```python
from build123d import *

# Parameters (mm, degrees)
SKETCH2_R           = 13.5
BOSS_EXTRUDE2_DEPTH = 10
CUT_EXTRUDE1_DEPTH  = 59.489315264
BOSS_EXTRUDE3_DEPTH = 10
SKETCH5_R           = 1.7
CUT_EXTRUDE3_DEPTH  = 59.489315264


with BuildPart() as part:
    # Sketch2 → Boss-Extrude2 (new body)
    # profile 1 of 4: a face of its own
    with BuildSketch(Plane(origin=(0, 0, 0), x_dir=(1, 0, 0), z_dir=(0, 1, 0))):
        with BuildLine():
            ThreePointArc((4.652086817, 15.830606061), (3.552193091, 19.577649142), (0, 21.2))
            ThreePointArc((0, 21.2), (-3.552193091, 19.577649142), (-4.652086817, 15.830606061))
            ThreePointArc((-4.652086817, 15.830606061), (-3.188214551, 16.189048396), (-1.697742762, 16.412424242))
            ThreePointArc((-1.697742762, 16.412424242), (-0.043802421, 18.199435597), (1.7, 16.5))
            ThreePointArc((1.7, 16.5), (1.699435597, 16.456197579), (1.697742762, 16.412424242))
            ThreePointArc((1.697742762, 16.412424242), (3.188214551, 16.189048396), (4.652086817, 15.830606061))
        make_face()
    # profile 2 of 4: a face of its own
    with BuildSketch(Plane(origin=(0, 0, 0), x_dir=(1, 0, 0), z_dir=(0, 1, 0))):
        with BuildLine():
            ThreePointArc((-1.697742762, 16.412424242), (-3.188214551, 16.189048396), (-4.652086817, 15.830606061))
            ThreePointArc((-4.652086817, 15.830606061), (-16.5, 0), (-4.652086817, -15.830606061))
            ThreePointArc((-4.652086817, -15.830606061), (-3.188214551, -16.189048396), (-1.697742762, -16.412424242))
            ThreePointArc((-1.697742762, -16.412424242), (0, -14.8), (1.697742762, -16.412424242))
            ThreePointArc((1.697742762, -16.412424242), (3.188214551, -16.189048396), (4.652086817, -15.830606061))
            ThreePointArc((4.652086817, -15.830606061), (16.5, 0), (4.652086817, 15.830606061))
            ThreePointArc((4.652086817, 15.830606061), (3.188214551, 16.189048396), (1.697742762, 16.412424242))
            ThreePointArc((1.697742762, 16.412424242), (0, 14.8), (-1.697742762, 16.412424242))
        make_face()
        with Locations(Location((0, 0, 0), (0, 0, 270))):
            Circle(SKETCH2_R, mode=Mode.SUBTRACT)
    # profile 3 of 4: a face of its own
    with BuildSketch(Plane(origin=(0, 0, 0), x_dir=(1, 0, 0), z_dir=(0, 1, 0))):
        with BuildLine():
            ThreePointArc((-1.697742762, -16.412424242), (-3.188214551, -16.189048396), (-4.652086817, -15.830606061))
            ThreePointArc((-4.652086817, -15.830606061), (-3.552193091, -19.577649142), (0, -21.2))
            ThreePointArc((0, -21.2), (3.552193091, -19.577649142), (4.652086817, -15.830606061))
            ThreePointArc((4.652086817, -15.830606061), (3.188214551, -16.189048396), (1.697742762, -16.412424242))
            ThreePointArc((1.697742762, -16.412424242), (1.699435597, -16.456197579), (1.7, -16.5))
            ThreePointArc((1.7, -16.5), (-0.043802421, -18.199435597), (-1.697742762, -16.412424242))
        make_face()
    # profile 4 of 4: a face of its own
    with BuildSketch(Plane(origin=(0, 0, 0), x_dir=(1, 0, 0), z_dir=(0, 1, 0))):
        with BuildLine():
            Line((0, 36), (0, 21.2))
            ThreePointArc((0, 21.2), (3.552193091, 19.577649142), (4.652086817, 15.830606061))
            ThreePointArc((4.652086817, 15.830606061), (16.5, 0), (4.652086817, -15.830606061))
            ThreePointArc((4.652086817, -15.830606061), (3.552193091, -19.577649142), (0, -21.2))
            Line((0, -21.2), (0, -36))
            Line((0, -36), (45, -36))
            Line((45, -36), (45, 36))
            Line((45, 36), (0, 36))
        make_face()
    extrude(amount=BOSS_EXTRUDE2_DEPTH)

    # Sketch3 → Cut-Extrude1 (cut, through all)
    with BuildSketch(Plane(origin=(0, 10, 0), x_dir=(1, 0, 0), z_dir=(0, 1, 0))):
        with BuildLine():
            Line((3, 16.22498074), (3, 33))
            Line((3, 33), (42, 33))
            Line((42, 33), (42, -33))
            Line((42, -33), (3, -33))
            Line((3, -33), (3, -16.22498074))
            ThreePointArc((3, -16.22498074), (16.5, 0), (3, 16.22498074))
        make_face()
    extrude(amount=-CUT_EXTRUDE1_DEPTH, mode=Mode.SUBTRACT)

    # Sketch4 → Boss-Extrude3 (add, through all)
    with BuildSketch(Plane(origin=(0, 10, 0), x_dir=(1, 0, 0), z_dir=(0, 1, 0))):
        with BuildLine():
            Line((37, -33), (42, -33))
            Line((42, -33), (42, -28))
            ThreePointArc((42, -28), (38.464466094, -29.464466094), (37, -33))
        make_face()
        with BuildLine():
            Line((37, 33), (42, 33))
            Line((42, 33), (42, 28))
            ThreePointArc((42, 28), (38.464466094, 29.464466094), (37, 33))
        make_face()
    extrude(amount=-BOSS_EXTRUDE3_DEPTH)

    # Sketch5 → Cut-Extrude3 (cut, through all)
    with BuildSketch(Plane(origin=(0, 10, 0), x_dir=(1, 0, 0), z_dir=(0, 1, 0))):
        with Locations(Location((42, 33, 0), (0, 0, 270))):
            Circle(SKETCH5_R)
        with Locations(Location((42, -33, 0), (0, 0, 270))):
            Circle(SKETCH5_R)
    extrude(amount=-CUT_EXTRUDE3_DEPTH, mode=Mode.SUBTRACT)


solid = part.part
```
Verification items for the finished model (mm, model axes). A direction names the side the tool comes from. Coordinates: 2 decimals unless noted, no trailing zeros. Order: outer loops, then holes, each group sorted by start corner. A loop starts at its lowest first (then second) coordinate and runs counter-clockwise, first axis right, second up. Notation, with made-up numbers: (-2.75, -18.75) -> (26.25, -18.75) arc R13 cw to (26.25, -11.75) -> close; hole circle Ø1 at (9.25, -5.5). An arc over 180 degrees is marked (long way). Put each result on its own line as item: value. Start each with the question number.
1) Cross-section at D-D (z = 8). Enter the section's corners in (x, y), plus the area to 3 significant figures.
2) Cross-section at A-A (z = 0). Enter the section's corners in (x, y).
3) Cross-section at C-C (y = 2.25). Enter the section's corners in (x, z), plus the area to 3 significant figures.
4) Release check for a two-part mould opening along X. For faces 4 (the cylindrical face through (-13.18, 4.93, -2.93)), 5 (the flat face through (22, 5, 36)), 6 (the flat face through (3, 5, -24)), 7 (the flat face through (45, 5, 1)) record: pulls with the +X half, pulls with the -X half, needs draft (parallel to the pull), parting line crosses it, or undercut.
5) Material ranges on L1, parallel to X at y = 3.25, z = 25.5; L2, parallel to X at y = 0.5, z = -6; L3, parallel to X at y = 8.25, z = 2, recorded low to high.
6) Tool access check on faces 1 (the cylindrical face through (39, 5, -29)), 2 (the flat face through (0, 5, -29)), 3 (the flat face through (0, 5, 28)). Record the directions out of +Z, -Z, +X, -X, +Y, -Y that give a thin tool (end or side, any length) a straight path to the whole face; none if there is none.
7) Cross-section at B-B (z = 29). Enter the section's corners in (x, y).
Geometry check:
1. outline: (-14.43, 0) -> (-10.87, 0) -> (-10.87, 10) -> (-14.43, 10) -> close; (10.87, 0) -> (14.43, 0) -> (14.43, 10) -> (10.87, 10) -> close; (42, 0) -> (45, 0) -> (45, 10) -> (42, 10) -> close
1. area: 101 mm^2
2. outline: (-16.5, 0) -> (-13.5, 0) -> (-13.5, 10) -> (-16.5, 10) -> close; (13.5, 0) -> (16.5, 0) -> (16.5, 10) -> (13.5, 10) -> close; (42, 0) -> (45, 0) -> (45, 10) -> (42, 10) -> close
3. outline: (-4.65, -15.83) arc R4.7 ccw to (0, -21.2) -> (0, -36) -> (45, -36) -> (45, 36) -> (0, 36) -> (0, 21.2) arc R4.7 ccw to (-4.65, 15.83) arc R16.5 ccw to start; hole circle Ø27 at (0, 0); hole circle Ø3.4 at (0, -16.5); hole circle Ø3.4 at (0, 16.5); hole (3, -33) -> (37, -33) arc R5 cw to (42, -28) -> (42, 28) arc R5 cw to (37, 33) -> (3, 33) -> (3, 16.22) arc R16.5 cw to (3, -16.22) -> close; hole circle Ø3.4 at (42, -33); hole circle Ø3.4 at (42, 33)
3. area: 890 mm^2
4. face 4: undercut
4. face 5: needs draft
4. face 6: undercut
4. face 7: pulls with the +X half
5. L1: x = 0 to 3, 42 to 45
5. L2: x = -15.37 to -12.09, 12.09 to 15.37, 42 to 45
5. L3: x = -16.38 to -13.35, 13.35 to 16.38, 42 to 45
6. face 1: +Y, -Y
6. face 2: -Z, -X, +Y, -Y
6. face 3: +Z, -X, +Y, -Y
7. outline: (0, 0) -> (3, 0) -> (3, 10) -> (0, 10) -> close; (39, 0) -> (45, 0) -> (45, 10) -> (39, 10) -> close
